For this review, use the dimensioned drawing (mm, ordinates from the lowest corner) and the shaded views. A direction names the side the tool comes from. Coordinates: 2 decimals unless noted, no trailing zeros. Loops run counter-clockwise (first coordinate to the right, second up) from the corner with the lowest first, then second, coordinate; pieces in that order, holes last. Notation, with made-up numbers: M 22,18.25 L 39,18.25 A20 cw 39,23.25 Z; hole C -7,86.5 d11. An arc over 180 degrees is marked long. Write item = value, one per line.
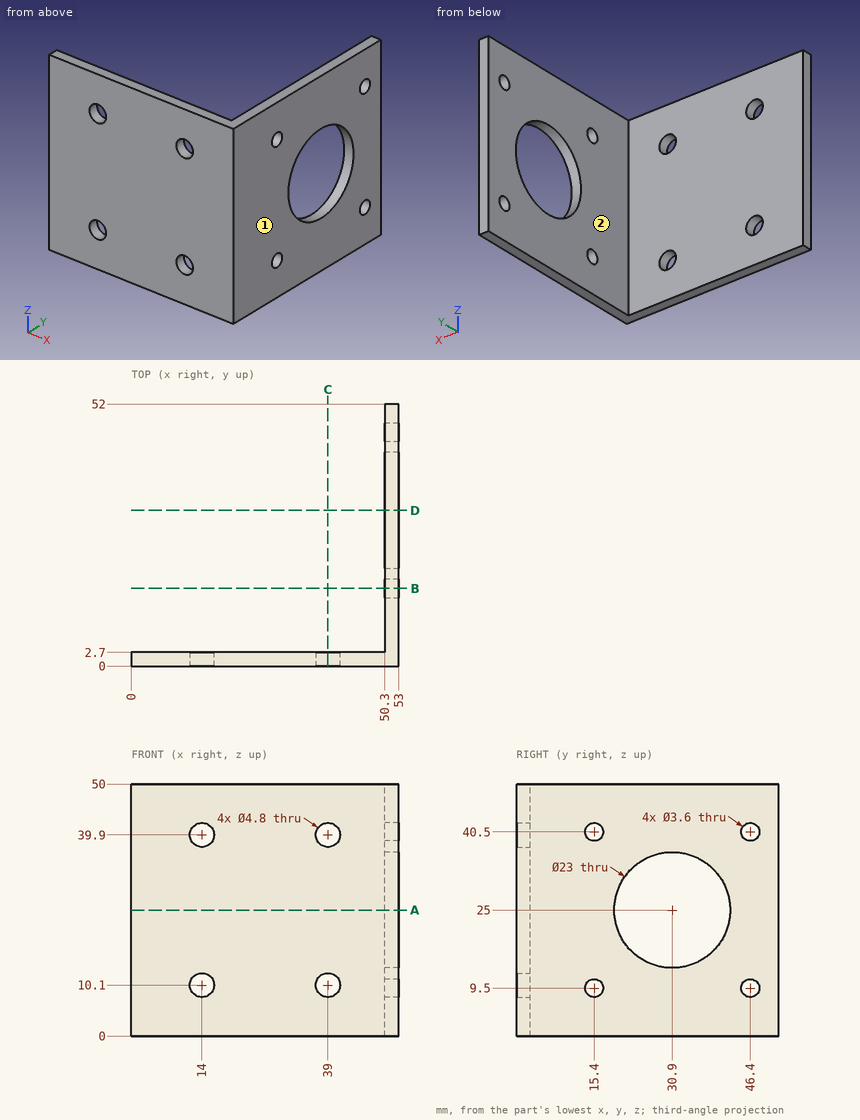
Q1. Add section B-B (y = 15.4). Write out the cut boundary in (x, z).
Solved:
outline = M 50.3,0 L 53,0 L 53,7.7 L 50.3,7.7 Z; M 50.3,11.3 L 53,11.3 L 53,38.7 L 50.3,38.7 Z; M 50.3,42.3 L 53,42.3 L 53,50 L 50.3,50 Z
Q2. Add section A-A (z = 25). Write out the cut boundary in (x, y).
Solved:
outline = M 0,0 L 53,0 L 53,19.4 L 50.3,19.4 L 50.3,2.7 L 0,2.7 Z; M 50.3,42.4 L 53,42.4 L 53,52 L 50.3,52 Z
Q3. Machinability: for the marked faces 1 and 2, which of the approach directions +Z, -Z, +X, -X, +Y, -Y give a long, thin tool a straight path to every point of the face, cutting with its end or side? Answer none if there is none.
Solved:
face_1 = +Z, -Z, +X, +Y, -Y
face_2 = +Z, -Z, -X, +Y
Q4. For pin 1 Ø6 at (x, z) = (39, 10.1) entering from +Y; pin 2 Ø12 at (y, z) = (33.5, 42) entering from -X; pin 3 Ø10 at (x, y) = (17.5, 7) entering from +Z, all flat-tipped, find the tip position at first contact; note any pin that passes through.
Solved:
pin_1 = 2.7
pin_2 = 50.3
pin_3 = 50
Q5. Add section D-D (y = 30.9). Write out the cut boundary in (x, z).
Solved:
outline = M 50.3,0 L 53,0 L 53,13.5 L 50.3,13.5 Z; M 50.3,36.5 L 53,36.5 L 53,50 L 50.3,50 Z
Q6. Add section C-C (x = 39). Write out the cut boundary in (y, z).
Solved:
outline = M 0,0 L 2.7,0 L 2.7,7.7 L 0,7.7 Z; M 0,12.5 L 2.7,12.5 L 2.7,37.5 L 0,37.5 Z; M 0,42.3 L 2.7,42.3 L 2.7,50 L 0,50 Z
Q7. For line 1 along Z through (x, y) = (39, 0.95); line 2 along X through (y, z) = (2, 10); line 3 along Z through (x, y) = (51.1, 46.4), list the stretches that pass through material, from the lowest coordinate up.
Solved:
line_1 = 0 to 7.7, 12.5 to 37.5, 42.3 to 50
line_2 = 0 to 11.6, 16.4 to 36.6, 41.4 to 53
line_3 = 0 to 7.7, 11.3 to 38.7, 42.3 to 50
